from build123d import *

# Parameters (mm, degrees)
F0_W     = 112
F0_H     = 50
F1_DEPTH = 3
F0_W_2   = 118
F0_H_2   = 56
F2_DEPTH = 83
F3_W     = 48
F3_H     = 28
F3_R     = 2.5
F4_DEPTH = 3
F3_R_2   = 2
F5_DEPTH = 3
F6_DEPTH = 76.6
F7_W     = 24.463284
F7_H     = 15
F8_DEPTH = 53.2


with BuildPart() as f1:
    # F0 (on Top) → F1 (new body)
    with BuildSketch(Plane.XY):
        Rectangle(F0_W, F0_H)
    extrude(amount=F1_DEPTH)

    # F0 (on Top) → F2 (join)
    with BuildSketch(Plane.XY):
        Rectangle(F0_W_2, F0_H_2)
        Rectangle(F0_W, F0_H, mode=Mode.SUBTRACT)
    extrude(amount=F2_DEPTH)

    # F3 (on face) → F4 (cut)
    with BuildSketch(Plane.XZ.offset(28)):
        with Locations((0, 30.5)):
            Rectangle(F3_W, F3_H)
        with Locations((0, 30.5)):
            Circle(F3_R, mode=Mode.SUBTRACT)
        with Locations((0, 30.5)):
            Circle(F3_R)
    extrude(amount=-F4_DEPTH, mode=Mode.SUBTRACT)

    # F3 (on face) → F5 (cut)
    with BuildSketch(Plane.XZ.offset(28)):
        with Locations((0, 50)):
            Circle(F3_R_2)
        with Locations((0, 11)):
            Circle(F3_R_2)
    extrude(amount=-F5_DEPTH, mode=Mode.SUBTRACT)

    # F3 (on face) → F6 (cut)
    with BuildSketch(Plane.XZ.offset(28)):
        with Locations((0, 30.5)):
            Circle(F3_R)
    extrude(amount=-F6_DEPTH, mode=Mode.SUBTRACT)

    # F7 (on face) → F8 (join)
    with BuildSketch(Plane.XY.offset(3)):
        with Locations((-39.3574, -17.5)):
            Rectangle(F7_W, F7_H)
        with Locations((39.3574, -17.5)):
            Rectangle(F7_W, F7_H)
    extrude(amount=F8_DEPTH)


solid = f1.part
Design review of the part built by this model. Coordinates are the model's own, in mm. A direction names the side the tool comes from. Give positions to 0.01 mm unless a question says otherwise; leave off trailing zeros. Order: outer loops, then holes, each group sorted by start corner. A loop starts at its lowest first (then second) coordinate and runs counter-clockwise, first axis right, second up. Notation, with made-up numbers: (55.25, -38.5) - (77.25, -38.5) arc R22 ccw to (77.25, -20.5) - close; hole circle Ø6 at (-3, 62.25). An arc over 180 degrees is marked (long way). Write item = value, one per line. Start each with the question number.
Q1. Tool access review of faces 4 (the face through (0, -27, 13)), 5 (the face through (39, -17, 56.2)), 6 (the face through (1.34, 26.48, 32.61)): name each direction out of +Z, -Z, +X, -X, +Y, -Y from which nothing blocks a thin tool from reaching the whole face with its end or side.
Q2. Clearance check with flat-ended pins moving along their axes: pin 1 Ø3 at (x, z) = (0, 50) entering from -Y; pin 2 Ø10 at (x, y) = (-46, -4) entering from +Z; pin 3 Ø4.5 at (x, y) = (-37.5, -21) entering from +Z. State where each tip first meets the part, or that it passes through.
Q3. We need section C-C on y = -5. State the section outline as (x, z) points.
Q4. Mouldability with a two-part tool opening along X and no side actions: class faces 1 (the face through (59, 0, 41)), 2 (the face through (-1, 28, 41)), 3 (the face through (24, -27, 30)) as released by +X, released by -X, zero draft, split by the parting line, or undercut.
Q5. We need section B-B on z = 30.5. State the section outline as (x, y) points, plus the area to 3 significant figures.
Q6. To check wall thickness, follow L1, parallel to Z at x = 0, y = -27; L2, parallel to X at y = -14.5, z = 16; L3, parallel to Y at x = 51.5, z = 30. State the ranges of each line that lie inside material, in increasing order. Write a range as from..to.
Q7. We need section A-A on x = 0. State the section outline as (y, z) points.
Q8. We need section D-D on x = -15.5. State the section outline as (y, z) points, plus the area to 3 significant figures.
Working result:
q1.face_4 = -Y
q1.face_5 = +Z
q1.face_6 = +Y, -Y
q2.pin_1 = 25
q2.pin_2 = 3
q2.pin_3 = 56.2
q3.outline = (-59, 0) - (59, 0) - (59, 83) - (56, 83) - (56, 3) - (-56, 3) - (-56, 83) - (-59, 83) - close
q4.face_1 = released by +X
q4.face_2 = zero draft
q4.face_3 = undercut
q5.outline = (-59, -28) - (-24, -28) - (-24, -25) - (-27.13, -25) - (-27.13, -10) - (-51.59, -10) - (-51.59, -25) - (-56, -25) - (-56, 25) - (-2.5, 25) - (-2.5, 28) - (-59, 28) - close; (2.5, 25) - (56, 25) - (56, -25) - (51.59, -25) - (51.59, -10) - (27.13, -10) - (27.13, -25) - (24, -25) - (24, -28) - (59, -28) - (59, 28) - (2.5, 28) - close
q5.area = 1,580 mm²
q6.L1 = 0..9, 13..16.5, 44.5..48, 52..83
q6.L2 = -59..-56, -51.59..-27.13, 27.13..51.59, 56..59
q6.L3 = -28..-10, 25..28
q7.outline = (-28, 0) - (28, 0) - (28, 28) - (25, 28) - (25, 3) - (-25, 3) - (-25, 9) - (-28, 9) - close; (-28, 13) - (-25, 13) - (-25, 16.5) - (-28, 16.5) - close; (-28, 44.5) - (-25, 44.5) - (-25, 48) - (-28, 48) - close; (-28, 52) - (-25, 52) - (-25, 83) - (-28, 83) - close; (25, 33) - (28, 33) - (28, 83) - (25, 83) - close
q8.outline = (-28, 0) - (28, 0) - (28, 83) - (25, 83) - (25, 3) - (-25, 3) - (-25, 16.5) - (-28, 16.5) - close; (-28, 44.5) - (-25, 44.5) - (-25, 83) - (-28, 83) - close
q8.area = 564 mm²
